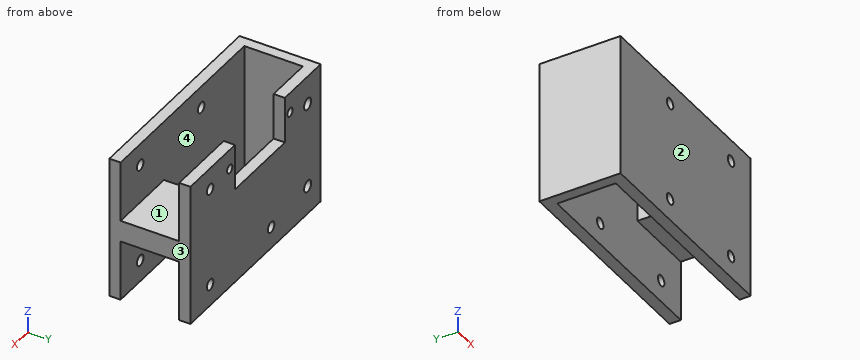
```python
from build123d import *

# Parameters (mm, degrees)
SKETCH1_W                 = 60
SKETCH1_H                 = 40
BOSS_EXTRUDE1_DEPTH       = 3.15
BOSS_EXTRUDE2_START       = 16.4
SKETCH1_2_W               = 60
SKETCH1_2_H               = 40
BOSS_EXTRUDE2_DEPTH       = 3.15
SKETCH2_W                 = 3
SKETCH2_H                 = 40
SKETCH2_W_2               = 20
SKETCH2_H_2               = 6
BOSS_EXTRUDE3_DEPTH       = 16.4
M2_CLEARANCE_HOLE1_D      = 2.4
M2_CLEARANCE_HOLE1_DEPTH  = 5
M2_CLEARANCE_HOLE1_TIP    = 0.721032743
F_3_0MM_DOWEL_HOLE1_D     = 3
SKETCH5_W                 = 23
SKETCH5_H                 = 13
CUT_EXTRUDE1_DEPTH        = 7
F_4_CLEARANCE_HOLE2_D     = 3.2639
F_4_CLEARANCE_HOLE2_DEPTH = 10
F_4_CLEARANCE_HOLE2_TIP   = 0.980574487


with BuildPart() as part:
    # Sketch1 → Boss-Extrude1 (new body)
    with BuildSketch(Plane(origin=(0, 0, 0), x_dir=(1, 0, 0), z_dir=(0, 1, 0))):
        with Locations((30, 0)):
            Rectangle(SKETCH1_W, SKETCH1_H)
    extrude(amount=-BOSS_EXTRUDE1_DEPTH)



with BuildPart() as body_2:
    # Sketch1<2> → Boss-Extrude2 (new body)
    with BuildSketch(Plane(origin=(0, 0, 0), x_dir=(1, 0, 0), z_dir=(0, 1, 0)).offset(BOSS_EXTRUDE2_START)):
        with Locations((30, 0)):
            Rectangle(SKETCH1_2_W, SKETCH1_2_H)
    extrude(amount=BOSS_EXTRUDE2_DEPTH)


with BuildPart() as part_1:
    add(part.part)

    add(body_2.part)  # Boss-Extrude3 merges body 2
    # Sketch2 → Boss-Extrude3 (add)
    with BuildSketch(Plane(origin=(0, 0, 0), x_dir=(1, 0, 0), z_dir=(0, 1, 0))):
        with Locations((1.5, 0)):
            Rectangle(SKETCH2_W, SKETCH2_H)
        with Locations((50, 0)):
            Rectangle(SKETCH2_W_2, SKETCH2_H_2)
    extrude(amount=BOSS_EXTRUDE3_DEPTH)

    # M2 Clearance Hole1
    with Locations(Plane(origin=(0, 19.55, 0), x_dir=(1, 0, 0), z_dir=(0, 1, 0))):
        with Locations((14.1, -14.4), (41.9, -14.4)):
            Hole(M2_CLEARANCE_HOLE1_D / 2, depth=M2_CLEARANCE_HOLE1_DEPTH)
            with Locations((0, 0, -(M2_CLEARANCE_HOLE1_DEPTH + M2_CLEARANCE_HOLE1_TIP / 2))):  # 118° drill point
                Cone(0, M2_CLEARANCE_HOLE1_D / 2, M2_CLEARANCE_HOLE1_TIP, mode=Mode.SUBTRACT)

    # Ø3.0mm Dowel Hole1 (through all)
    with Locations(Plane(origin=(0, 19.55, 0), x_dir=(1, 0, 0), z_dir=(0, 1, 0))):
        with Locations((50.95, -13.9), (22.85, 13.9), (50.95, 13.9), (22.85, -13.9)):
            Hole(F_3_0MM_DOWEL_HOLE1_D / 2)

    # Sketch5 → Cut-Extrude1 (cut)
    with BuildSketch(Plane(origin=(0, 19.55, 0), x_dir=(1, 0, 0), z_dir=(0, 1, 0))):
        with Locations((28, -13.5)):
            Rectangle(SKETCH5_W, SKETCH5_H)
    extrude(amount=-CUT_EXTRUDE1_DEPTH, mode=Mode.SUBTRACT)

    # #4 Clearance Hole2
    with Locations(Plane(origin=(0, 19.55, 0), x_dir=(1, 0, 0), z_dir=(0, 1, 0))):
        with Locations((6, 12), (6, -12)):
            Hole(F_4_CLEARANCE_HOLE2_D / 2, depth=F_4_CLEARANCE_HOLE2_DEPTH)
            with Locations((0, 0, -(F_4_CLEARANCE_HOLE2_DEPTH + F_4_CLEARANCE_HOLE2_TIP / 2))):  # 118° drill point
                Cone(0, F_4_CLEARANCE_HOLE2_D / 2, F_4_CLEARANCE_HOLE2_TIP, mode=Mode.SUBTRACT)


solid = part_1.part
```
Can you work these out from the model? Positions are in its coordinate system, mm. Face numbers are marked on the shaded views. Give positions to 0.01 mm unless a question says otherwise; leave off trailing zeros. Loops run counter-clockwise (first coordinate to the right, second up) from the corner with the lowest first, then second, coordinate; pieces in that order, holes last. Notation, with made-up numbers: M 26.5,45 L 59.5,45 A22 ccw 59.5,82 Z; hole C -4.75,25 d1. An arc over 180 degrees is marked long. Use one line per item in the form item = value. Start each with the question number.
(1) I want a section at A-A, the plane z = 18. Write out the boundary of the cut face in (x, y), and give its area (3 significant figures).
(2) I'm going to push flat-ended pins straight in: P1, Ø1.8, axis at y = 8.5, z = -0.5, coming from the -X side; P2, Ø2, axis at x = 44.5, y = 2, coming from the -Z side; P3, Ø1.8, axis at x = 50.95, z = -13.9, coming from the +Y side; P4, Ø5, axis at y = 8, z = 12.5, coming from the +X side. Where does each tip first touch, or does it pass through?
(3) Please list where these lines run through material, in increasing order: line 1 (X direction, y = 18.8, z = -13.9); line 2 (Z direction, x = 22.85, y = -0.85); line 3 (Z direction, x = 6, y = 18.2).
(4) I want a section at B-B, the plane x = 6. Write out the boundary of the cut face in (y, z).
(5) Thinking about a two-plate mould opening in Y: for the marked faces 1, 2, 3 and 4, which applies, released by +Y, released by -Y, zero draft, split by the parting line, or undercut?
(6) I want a section at C-C, the plane y = 6.25. Write out the boundary of the cut face in (x, z), and give its area (3 significant figures).
(7) I want a section at D-D, the plane x = 41.9. Write out the boundary of the cut face in (y, z).
Worked out:
q1.outline = M 0,-3.15 L 60,-3.15 L 60,0 L 3,0 L 3,16.4 L 16.5,16.4 L 16.5,19.55 L 0,19.55 Z; M 39.5,16.4 L 60,16.4 L 60,19.55 L 39.5,19.55 Z
q1.area = 355 mm²
q2.P1 = 0
q2.P2 = -3
q2.P3 = through
q2.P4 = 3
q3.line_1 = 0 to 21.35, 24.35 to 49.45, 52.45 to 60
q3.line_2 = -20 to -15.4, -12.4 to 12.4, 15.4 to 20
q3.line_3 = -20 to -13.63, -10.37 to 10.37, 13.63 to 20
q4.outline = M -3.15,-20 L 0,-20 L 0,20 L -3.15,20 Z; M 16.4,-20 L 19.55,-20 L 19.55,-13.63 L 16.4,-13.63 Z; M 16.4,-10.37 L 19.55,-10.37 L 19.55,10.37 L 16.4,10.37 Z; M 16.4,13.63 L 19.55,13.63 L 19.55,20 L 16.4,20 Z
q5.face_1 = undercut
q5.face_2 = released by -Y
q5.face_3 = zero draft
q5.face_4 = undercut
q6.outline = M 0,-20 L 3,-20 L 3,20 L 0,20 Z; M 40,-3 L 60,-3 L 60,3 L 40,3 Z
q6.area = 240 mm²
q7.outline = M -3.15,-20 L 0,-20 L 0,-3 L 16.4,-3 L 16.4,-20 L 19.55,-20 L 19.55,13.2 L 16.4,13.2 L 16.4,3 L 0,3 L 0,20 L -3.15,20 Z; M 16.4,15.6 L 19.55,15.6 L 19.55,20 L 16.4,20 Z
